Build history of the part. All positions in model axes, mm. Give positions to 0.01 mm unless a question says otherwise; leave off trailing zeros. Order: outer loops, then holes, each group sorted by start corner. A loop starts at its lowest first (then second) coordinate and runs counter-clockwise, first axis right, second up. Notation, with made-up numbers: (65.5, 80.5) - (120.5, 80.5) arc R35 cw to (120.5, 112.5) - close; hole circle Ø6 at (87.5, 53). An arc over 180 degrees is marked (long way). Use a Markdown table: item, result.
from build123d import *

# Parameters (mm, degrees)
SKETCH2_R           = 0.79375
SKETCH2_R_2         = 1.2065
BOSS_EXTRUDE1_DEPTH = 1.6


with BuildPart() as part:
    # Sketch2 → Boss-Extrude1 (new body)
    with BuildSketch(Plane(origin=(0, 0, 0), x_dir=(1, 0, 0), z_dir=(0, 1, 0))):
        with BuildLine():
            Line((-1.5875, 48.732377473), (-1.5875, 50.912554448))
            ThreePointArc((-1.5875, 50.912554448), (-2.405542288, 52.779761356), (-4.332745385, 53.444248412))
            ThreePointArc((-4.332745385, 53.444248412), (-35.306836043, 40.354525144), (-52.395068561, 11.393733429))
            ThreePointArc((-52.395068561, 11.393733429), (-52.305343014, 10.000391507), (-51.492756078, 8.864981951))
            ThreePointArc((-51.492756078, 8.864981951), (-47.415865481, 7.171089887), (-43.058200955, 7.878950847))
            ThreePointArc((-43.058200955, 7.878950847), (-40.630358405, 7.324125051), (-40.580789574, 4.834186489))
            ThreePointArc((-40.580789574, 4.834186489), (-42.191393903, 0), (-40.580789574, -4.834186489))
            ThreePointArc((-40.580789574, -4.834186489), (-40.630358405, -7.324125051), (-43.058200955, -7.878950847))
            ThreePointArc((-43.058200955, -7.878950847), (-47.415865481, -7.171089887), (-51.492756078, -8.864981951))
            ThreePointArc((-51.492756078, -8.864981951), (-52.305343014, -10.000391507), (-52.395068561, -11.393733429))
            ThreePointArc((-52.395068561, -11.393733429), (-35.306836043, -40.354525144), (-4.332745385, -53.444248412))
            ThreePointArc((-4.332745385, -53.444248412), (-2.405542288, -52.779761356), (-1.5875, -50.912554448))
            Line((-1.5875, -50.912554448), (-1.5875, -48.732377473))
            ThreePointArc((-1.5875, -48.732377473), (-2.077855675, -47.232191438), (-3.359593023, -46.311237478))
            ThreePointArc((-3.359593023, -46.311237478), (-8.418901259, -42.972008429), (-10.972940557, -37.474378601))
            ThreePointArc((-10.972940557, -37.474378601), (-11.900363007, -36.272469223), (-13.41319791, -36.399075336))
            ThreePointArc((-13.41319791, -36.399075336), (-24.083249547, -33.474502145), (-19.817234122, -23.266454208))
            ThreePointArc((-19.817234122, -23.266454208), (-18.773073396, -22.097738961), (-19.241161334, -20.602058302))
            ThreePointArc((-19.241161334, -20.602058302), (-28.189840294, 0), (-19.241161334, 20.602058302))
            ThreePointArc((-19.241161334, 20.602058302), (-18.773073396, 22.097738961), (-19.817234122, 23.266454208))
            ThreePointArc((-19.817234122, 23.266454208), (-24.083249547, 33.474502145), (-13.41319791, 36.399075336))
            ThreePointArc((-13.41319791, 36.399075336), (-11.900363007, 36.272469223), (-10.972940557, 37.474378601))
            ThreePointArc((-10.972940557, 37.474378601), (-8.418901259, 42.972008429), (-3.359593023, 46.311237478))
            ThreePointArc((-3.359593023, 46.311237478), (-2.077855675, 47.232191438), (-1.5875, 48.732377473))
        make_face()
        with Locations(Location((-39.125436229, 29.324414144, 0), (0, 0, 270))):
            Circle(SKETCH2_R, mode=Mode.SUBTRACT)
        with Locations(Location((-30.283799979, -15.742734369, 0), (0, 0, 270))):
            Circle(SKETCH2_R, mode=Mode.SUBTRACT)
        with Locations(Location((-46.479977899, -15.176715045, 0), (0, 0, 270))):
            Circle(SKETCH2_R, mode=Mode.SUBTRACT)
        with Locations(Location((-34.13125, 0, 0), (0, 0, 270))):
            Circle(SKETCH2_R, mode=Mode.SUBTRACT)
        with Locations(Location((-46.479977899, 15.176715045, 0), (0, 0, 270))):
            Circle(SKETCH2_R, mode=Mode.SUBTRACT)
        with Locations(Location((-30.283799979, 15.742734369, 0), (0, 0, 270))):
            Circle(SKETCH2_R, mode=Mode.SUBTRACT)
        with Locations(Location((-38.167598541, -9.327981047, 0), (0, 0, 270))):
            Circle(SKETCH2_R_2, mode=Mode.SUBTRACT)
        with Locations(Location((-38.167598541, 9.327981047, 0), (0, 0, 270))):
            Circle(SKETCH2_R_2, mode=Mode.SUBTRACT)
        with Locations(Location((-26.788483085, 27.092197659, 0), (0, 0, 270))):
            Circle(SKETCH2_R_2, mode=Mode.SUBTRACT)
        with Locations(Location((-27.610010923, 40.353541627, 0), (0, 0, 270))):
            Circle(SKETCH2_R, mode=Mode.SUBTRACT)
        with Locations(Location((-39.125436229, -29.324414144, 0), (0, 0, 270))):
            Circle(SKETCH2_R, mode=Mode.SUBTRACT)
        with Locations(Location((-26.788483085, -27.092197659, 0), (0, 0, 270))):
            Circle(SKETCH2_R_2, mode=Mode.SUBTRACT)
        with Locations(Location((-27.610010923, -40.353541627, 0), (0, 0, 270))):
            Circle(SKETCH2_R, mode=Mode.SUBTRACT)
    extrude(amount=BOSS_EXTRUDE1_DEPTH)


solid = part.part
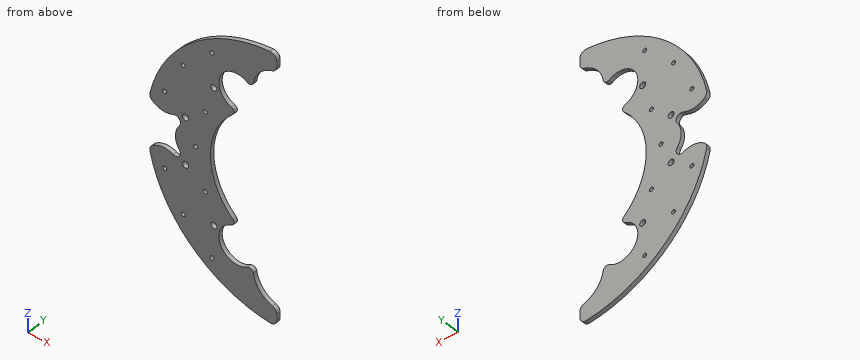
1) Slice it at A-A (x = -8). Write the cut outline in (y, z).
Computed:
| item | result |
|---|---|
| outline | (0, -53.02) - (1.6, -53.02) - (1.6, -43.43) - (0, -43.43) - close; (0, 43.43) - (1.6, 43.43) - (1.6, 53.02) - (0, 53.02) - close |
2) Slice it at D-D (x = -36). Write the cut outline in (y, z).
Computed:
| item | result |
|---|---|
| outline | (0, -39.74) - (1.6, -39.74) - (1.6, 39.74) - (0, 39.74) - close |
3) Slice it at C-C (z = -24.5). Write the cut outline in (x, y), and give its area (3 significant figures).
Computed:
| item | result |
|---|---|
| outline | (-47.69, 0) - (-22.07, 0) - (-22.07, 1.6) - (-47.69, 1.6) - close |
| area | 41.0 mm² |
4) Wall check: line 1 (Z direction, x = -22, y = 0.95); line 2 (X direction, y = 0.55, z = 0) (1 decimal); line 3 (Z direction, x = -21.5, y = 1.15). Give the ranges that are in metal, low to high. Write a range as from..to.
Computed:
| item | result |
|---|---|
| line 1 | z = -48.9..-36.05, -24.44..-17.63, 17.63..24.44, 36.05..48.9 |
| line 2 | x = -42.2..-34.9, -33.3..-28.2 |
| line 3 | z = -49.12..-36.41, -24.09..-18.23, 18.23..24.09, 36.41..49.12 |
5) Slice it at B-B (y = 1.35). State how many separate pieces and enclosed holes the cut face has, and give its area (3 significant figures).
Computed:
| item | result |
|---|---|
| separate pieces | 1 |
| enclosed holes | 13 |
| area | 2,300 mm² |
